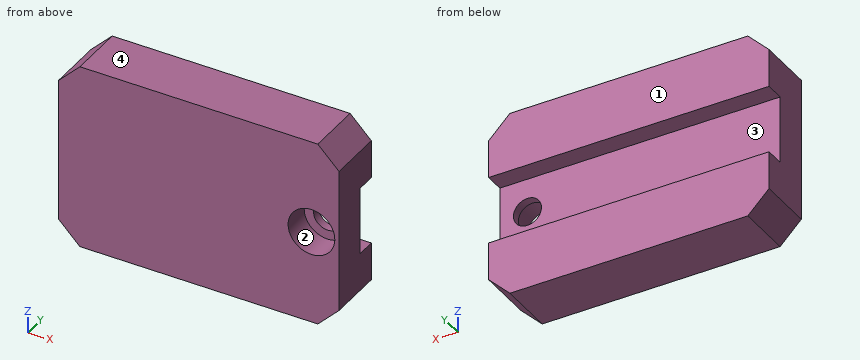
```python
from build123d import *

# Parameters (mm, degrees)
ESBO_O1_W                = 66
ESBO_O1_H                = 13
RESSALTO_EXTRUS_O1_DEPTH = 44
ESBO_O2_W                = 66
ESBO_O2_H                = 16
CORTE_EXTRUS_O1_DEPTH    = 4.5
CHANFRO1_SIZE            = 5
ESBO_O4_R                = 3.3
CORTE_EXTRUS_O2_DEPTH    = 2
ESBO_O5_R                = 5.5
CORTE_EXTRUS_O3_DEPTH    = 6.5


with BuildPart() as part:
    # Esboço1 → Ressalto-extrusão1 (new body)
    with BuildSketch(Plane.XY):
        with Locations((33, -6.5)):
            Rectangle(ESBO_O1_W, ESBO_O1_H)
    extrude(amount=RESSALTO_EXTRUS_O1_DEPTH)

    # Esboço2 → Corte-extrusão1 (cut)
    with BuildSketch(Plane(origin=(0, 0, 0), x_dir=(1, 0, 0), z_dir=(0, 1, 0))):
        with Locations((33, -22)):
            Rectangle(ESBO_O2_W, ESBO_O2_H)
    extrude(amount=-CORTE_EXTRUS_O1_DEPTH, mode=Mode.SUBTRACT)

    # Chanfro1
    chanfro1_edges = [part.edges().sort_by_distance(p)[0] for p in [
        (66, -6.5, 44),
        (0, -6.5, 44),
        (66, -6.5, 0),
        (0, -6.5, 0),
    ]]
    chamfer(chanfro1_edges, length=CHANFRO1_SIZE)

    # Esboço4 → Corte-extrusão2 (cut)
    with BuildSketch(Plane(origin=(0, -4.5, 0), x_dir=(1, 0, 0), z_dir=(0, 1, 0))):
        with Locations(Location((59.5, -22, 0), (0, 0, 270))):
            Circle(ESBO_O4_R)
    extrude(amount=-CORTE_EXTRUS_O2_DEPTH, mode=Mode.SUBTRACT)

    # Esboço5 → Corte-extrusão3 (cut)
    with BuildSketch(Plane.XZ.offset(13)):
        with Locations(Location((59.5, 22, 0), (0, 0, 270))):
            Circle(ESBO_O5_R)
    extrude(amount=-CORTE_EXTRUS_O3_DEPTH, mode=Mode.SUBTRACT)


solid = part.part
```
Geometry check sheet. Reference: the model listing, model coordinates, mm. Face numbers are marked on the shaded views. Coordinates: 2 decimals unless noted, no trailing zeros. Order: outer loops, then holes, each group sorted by start corner. A loop starts at its lowest first (then second) coordinate and runs counter-clockwise, first axis right, second up. Notation, with made-up numbers: M -28,-37 L -23,-37 A16 cw -23,-23 Z; hole C 71,46.25 d2. An arc over 180 degrees is marked long. Answer as a JSON object with one key per item and string values.
Q1. Depth check by flat-ended pin: pin 1 Ø6 at (x, z) = (59.5, 22) entering from +Y; pin 2 Ø8 at (x, z) = (43.5, 19) entering from +Y. Enter the tip coordinate at first touch or a pass-through.
Results are:
{"pin 1": "passes through", "pin 2": "stops at y = -4.5"}
Q2. Release check for a two-part mould opening along Z. For the marked faces 1, 2, 3 and 4 record: released by +Z, released by -Z, zero draft, split by the parting line, or undercut.
Results are:
{"face 1": "zero draft", "face 2": "undercut", "face 3": "undercut", "face 4": "released by +Z"}
Q3. Cross-section at B-B on z = 22. Record the cut outline in (x, y).
Results are:
{"outline": "M 0,-13 L 54,-13 L 54,-6.5 L 56.2,-6.5 L 56.2,-4.5 L 0,-4.5 Z; M 62.8,-6.5 L 65,-6.5 L 65,-13 L 66,-13 L 66,-4.5 L 62.8,-4.5 Z"}
Q4. Cross-section at C-C on y = -1.25. Record the cut outline in (x, z).
Results are:
{"outline": "M 0,5 L 5,0 L 61,0 L 66,5 L 66,14 L 0,14 Z; M 0,30 L 66,30 L 66,39 L 61,44 L 5,44 L 0,39 Z"}
Q5. Cross-section at A-A on x = 59.5. Record the cut outline in (y, z), and give its area (3 significant figures).
Results are:
{"outline": "M -13,0 L 0,0 L 0,14 L -4.5,14 L -4.5,18.7 L -6.5,18.7 L -6.5,16.5 L -13,16.5 Z; M -13,27.5 L -6.5,27.5 L -6.5,25.3 L -4.5,25.3 L -4.5,30 L 0,30 L 0,44 L -13,44 Z", "area": "415 mm²"}
Q6. Cross-section at D-D on y = -10.25. Record the cut outline in (x, z), and give its area (3 significant figures).
Results are:
{"outline": "M 0,5 L 5,0 L 61,0 L 66,5 L 66,39 L 61,44 L 5,44 L 0,39 Z; hole C 59.5,22 d11", "area": "2,760 mm²"}
Q7. Scan lines: line 1 (Z direction, x = 15.5, y = -2); line 2 (X direction, y = -4.85, z = 22); line 3 (X direction, y = -11.5, z = 25). Record each from-to range of solid material in increasing order.
Results are:
{"line 1": "z = 0 to 14, 30 to 44", "line 2": "x = 0 to 56.2, 62.8 to 66", "line 3": "x = 0 to 54.89, 64.11 to 66"}
